from build123d import *

# Parameters (mm, degrees)
BASE_FLANGE1_DEPTH           = 0.7
SKETCH4_R                    = 1.5
SKETCH4_R_2                  = 3
CUT_EXTRUDE1_DEPTH           = 45.726837581
EDGE_FLANGE1_STRIP_W         = 4.2732
EDGE_FLANGE1_STRIP_H         = 0.7
EDGE_FLANGE1_STRIP_CUT_DEPTH = 30
EDGE_FLANGE1_DEPTH           = 30
SKETCH11_W                   = 9.2634
SKETCH11_H                   = 2.5
TAB1_DEPTH                   = 0.7
SKETCH10_R                   = 1.65
CUT_EXTRUDE2_DEPTH           = 0.7
BREAK_CORNER1_START          = -40.7
BREAK_CORNER1_DEPTH          = 0.7


# Read off the part's stored shape, not the designer's step: Break-Corner1
# Sheet-metal steps are written as plain solids
with BuildPart() as part:
    # Sketch1 → Base-Flange1 (new body)
    with BuildSketch(Plane(origin=(0, 0, 0), x_dir=(0, 0, -1), z_dir=(1, 0, 0))):
        with BuildLine():
            Line((-19.2, -5.6), (-15, -20))
            Line((-15, -20), (-15, -40))
            Line((-15, -40), (15, -40))
            Line((15, -40), (15, -20))
            Line((15, -20), (19.2, -5.6))
            ThreePointArc((19.2, -5.6), (0, 20), (-19.2, -5.6))
        make_face()
    extrude(amount=-BASE_FLANGE1_DEPTH)

    # Sketch4 → Cut-Extrude1 (cut, through all)
    with BuildSketch(Plane(origin=(0, 0, 0), x_dir=(0, 0, -1), z_dir=(1, 0, 0))):
        with Locations((-10.2108, 10)):
            Circle(SKETCH4_R)
        with Locations((10.2108, 10)):
            Circle(SKETCH4_R)
        with Locations((0, 10)):
            Circle(SKETCH4_R_2)
        with Locations((0, -12.1742)):
            Circle(SKETCH4_R)
    extrude(amount=-CUT_EXTRUDE1_DEPTH, mode=Mode.SUBTRACT)

    # Edge-Flange1 strip (across the edge) → Edge-Flange1 strip cut (cut)
    with BuildSketch(Plane(origin=(0, -40, 15), x_dir=(0, 1, 0), z_dir=(0, 0, -1))):
        with Locations((-1.4, -0.35)):
            Rectangle(EDGE_FLANGE1_STRIP_W, EDGE_FLANGE1_STRIP_H)
    extrude(amount=EDGE_FLANGE1_STRIP_CUT_DEPTH, mode=Mode.SUBTRACT)

    # Edge-Flange1 section (across the edge) → Edge-Flange1 (add)
    with BuildSketch(Plane(origin=(0, -40, 15), x_dir=(0, 1, 0), z_dir=(0, 0, -1))):
        with BuildLine():
            Line((-0.7, 0.7366), (-0.7, 10))
            Line((-0.7, 10), (0, 10))
            Line((0, 10), (0, 0.7366))
            ThreePointArc((0, 0.7366), (0.215745145, 0.215745145), (0.7366, 0))
            Line((0.7366, 0), (0.7366, -0.7))
            ThreePointArc((0.7366, -0.7), (-0.279229602, -0.279229602), (-0.7, 0.7366))
        make_face()
    extrude(amount=EDGE_FLANGE1_DEPTH)

    # Sketch11 → Tab1 (add)
    with BuildSketch(Plane(origin=(0, -40, 0), x_dir=(1, 0, 0), z_dir=(0, 1, 0))):
        with Locations((5.3683, -16.25)):
            Rectangle(SKETCH11_W, SKETCH11_H)
    tab1 = extrude(amount=-TAB1_DEPTH)

    # Mirror1: Tab1 across plane
    add(tab1.mirror(Plane.XY))

    # Sketch10 → Cut-Extrude2 (cut)
    with BuildSketch(Plane(origin=(0, -40, 0), x_dir=(1, 0, 0), z_dir=(0, 1, 0))):
        with Locations(Location((5, 10, 0), (0, 0, 180))):
            Circle(SKETCH10_R)
        with Locations((5, -10)):
            Circle(SKETCH10_R)
    extrude(amount=-CUT_EXTRUDE2_DEPTH, mode=Mode.SUBTRACT)

    # Break-Corner1 outline → Break-Corner1 (cut)
    with BuildSketch(Plane(origin=(0, 0, 0), x_dir=(1, 0, 0), z_dir=(0, 1, 0)).offset(BREAK_CORNER1_START)):
        with BuildLine():
            Line((10, -17.5), (10, -15))
            ThreePointArc((10, -15), (9.267766953, -16.767766953), (7.5, -17.5))
            Line((7.5, -17.5), (10, -17.5))
        make_face()
        with BuildLine():
            ThreePointArc((0.7366, 15), (1.468833047, 16.767766953), (3.2366, 17.5))
            Line((3.2366, 17.5), (0.7366, 17.5))
            Line((0.7366, 17.5), (0.7366, 15))
        make_face()
        with BuildLine():
            ThreePointArc((7.5, 17.5), (9.267766953, 16.767766953), (10, 15))
            Line((10, 15), (10, 17.5))
            Line((10, 17.5), (7.5, 17.5))
        make_face()
        with BuildLine():
            Line((0.7366, -17.5), (3.2366, -17.5))
            ThreePointArc((3.2366, -17.5), (1.468833047, -16.767766953), (0.7366, -15))
            Line((0.7366, -15), (0.7366, -17.5))
        make_face()
    extrude(amount=BREAK_CORNER1_DEPTH, mode=Mode.SUBTRACT)


solid = part.part
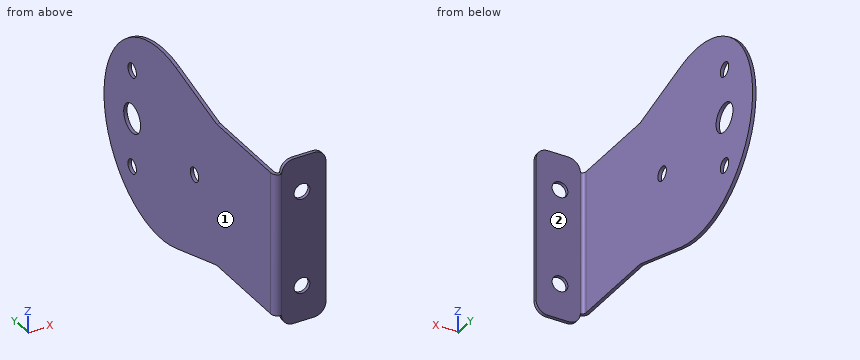
Model file for the job. Use its own axes, mm. Face numbers are marked on the shaded views. A direction names the side the tool comes from. Give positions to 0.01 mm unless a question says otherwise; leave off trailing zeros. Loops run counter-clockwise (first coordinate to the right, second up) from the corner with the lowest first, then second, coordinate; pieces in that order, holes last.
Item 1: Drill centre lines: line 1 along Z through (x, y) = (5, -40.4); line 2 along Y through (x, z) = (6, -5); line 3 along X through (y, z) = (11.5, 12). Where is each one in solid material? Low to high.
Check values:
line 1: z = -17.5 to -11.65, -8.35 to 8.35, 11.65 to 17.5
line 2: y = -40.7 to -40
line 3: x = -0.7 to 0
Item 2: Slice it at A-A (x = 5). Write the cut outline in (y, z), plus the area to 3 significant figures.
Check values:
outline: (-40.7, -17.5) - (-40, -17.5) - (-40, -11.65) - (-40.7, -11.65) - close; (-40.7, -8.35) - (-40, -8.35) - (-40, 8.35) - (-40.7, 8.35) - close; (-40.7, 11.65) - (-40, 11.65) - (-40, 17.5) - (-40.7, 17.5) - close
area: 19.9 mm2
Item 3: Slice it at D-D (z = 5). Write the cut outline in (x, y).
Check values:
outline: (-0.7, -39.26) arc R1.44 ccw to (0.74, -40.7) - (10, -40.7) - (10, -40) - (0.74, -40) arc R0.74 cw to (0, -39.26) - (0, 19.36) - (-0.7, 19.36) - close
Item 4: Which spindle directions (+Z, -Z, +X, -X, +Y, -Y) get a long thin tool onto all of the face, cutting with end or side? Do the marked faces 1 and 2. Say none if no direction does.
Check values:
face 1: +Z, -Z, -X, +Y, -Y
face 2: +Z, -Z, +X, +Y
Item 5: Drop flat-ended pins along their axis: P1, Ø3.5, axis at y = 10, z = -10.21, coming from the +X side; P2, Ø0.8, axis at x = 4.5, y = -40, coming from the +Z side; P3, Ø4.5, axis at x = 5, z = 10, coming from the +Y side. Give the stop position or say it passes through.
Check values:
P1: stops at x = 0
P2: stops at z = 17.5
P3: stops at y = -40
Item 6: Slice it at B-B (z = -10). Write the cut outline in (x, y), plus the area to 3 significant figures.
Check values:
outline: (-0.7, -39.26) arc R1.44 ccw to (0.74, -40.7) - (3.35, -40.7) - (3.35, -40) - (0.74, -40) arc R0.74 cw to (0, -39.26) - (0, 8.51) - (-0.7, 8.51) - close; (-0.7, 11.49) - (0, 11.49) - (0, 17.32) - (-0.7, 17.32) - close; (6.65, -40.7) - (10, -40.7) - (10, -40) - (6.65, -40) - close
area: 42.9 mm2
Item 7: Slice it at C-C (y = 10). Write the cut outline in (x, z), plus the area to 3 significant figures.
Check values:
outline: (-0.7, -17.32) - (0, -17.32) - (0, -11.71) - (-0.7, -11.71) - close; (-0.7, -8.71) - (0, -8.71) - (0, -3) - (-0.7, -3) - close; (-0.7, 3) - (0, 3) - (0, 8.71) - (-0.7, 8.71) - close; (-0.7, 11.71) - (0, 11.71) - (0, 17.32) - (-0.7, 17.32) - close
area: 15.8 mm2
